from build123d import *

# Parameters (mm, degrees)
F0_W     = 254
F0_H     = 177.8
F1_DEPTH = 1.5875
F2_W     = 1.058418
F2_H     = 63.5
F3_DEPTH = 25.4
F4_R     = 3.96875
F5_DEPTH = 12.7
F6_R     = 3.96875
F7_DEPTH = 12.7


with BuildPart() as f1:
    # F0 (on Top) → F1 (new body)
    with BuildSketch(Plane.XY):
        with Locations((29.202467, -74.189657)):
            Rectangle(F0_W, F0_H)
    extrude(amount=F1_DEPTH)

    # F2 (on face) → F3 (join)
    with BuildSketch(Plane.XY.offset(1.5875)):
        with Locations((118.058609, -74.189657)):
            Rectangle(F2_W, F2_H)
    extrude(amount=F3_DEPTH)

    # F4 (on face) → F5 (join)
    with BuildSketch(Plane.XY.offset(1.5875)):
        with Locations((-34.60809, -83.712486)):
            Circle(F4_R)
        with Locations((-34.8706, -67.839657)):
            Circle(F4_R)
    extrude(amount=F5_DEPTH)

    # F6 (on face) → F7 (join)
    with BuildSketch(Plane.XY.offset(1.5875)):
        with Locations((41.3294, -67.839657)):
            Circle(F6_R)
        with Locations((-34.297533, -151.180522)):
            Circle(F6_R)
    extrude(amount=F7_DEPTH)


solid = f1.part
Geometry: final body of the model. Coordinates: model frame, mm. A direction names the side the tool comes from. Coordinates: 2 decimals unless noted, no trailing zeros. Order: outer loops, then holes, each group sorted by start corner. A loop starts at its lowest first (then second) coordinate and runs counter-clockwise, first axis right, second up.
(1) Section query B-B (y = -55). Return the cut outline in (x, z), plus the area to 3 significant figures.
(2) First-contact query: pin 1 (6.5 mm diameter, centred on x = -35, y = -67, fed in from +Z); pin 2 (7.5 mm diameter, centred on y = -69.5, z = 12, fed in from +X); pin 3 (3 mm diameter, centred on y = -53, z = 21, fed in from -X). Flat tips, straight axial feed; report the tip coordinate or a pass-through.
(3) Material intervals for probe 1 along X at (y, z) = (-84.5, 19.5); probe 2 along Z at (x, y) = (0, -14), sorted ascending.
(4) Section query D-D (z = 18.25). Return the cut outline in (x, y), plus the area to 3 significant figures.
(5) Section query A-A (z = 5.5). Return the cut outline in (x, y), plus the area to 3 significant figures.
(6) Draft query along Y for faces 1 (the face through (40.469, -71.714, 7.849)), 2 (the face through (-37.447, -153.595, 7.849)), 3 (the face through (-34, -151, 14.288)). Return one class per face: pulls with the +Y half, pulls with the -Y half, needs draft (parallel to the pull), parting line crosses it, or undercut.
(7) Access query for faces 4 (the face through (41, -68, 14.288)), 5 (the face through (-35.731, -71.714, 7.849)), 6 (the face through (118.588, -75, 14)), 7 (the face through (117.529, -75, 14)), 8 (the face through (27, -73, 0)). Directions: +Z, -Z, +X, -X, +Y, -Y. A direction counts if a zero-diameter tool reaches every point of the face in a straight line with its end or side. Return the directions, or none.
(8) Section query C-C (x = -27). Return the cut outline in (y, z).
Solution:
1. outline: (-97.8, 0) - (156.2, 0) - (156.2, 1.59) - (118.59, 1.59) - (118.59, 26.99) - (117.53, 26.99) - (117.53, 1.59) - (-97.8, 1.59) - close
1. area: 430 mm2
2. pin 1: stops at z = 14.29
2. pin 2: stops at x = 118.59
2. pin 3: stops at x = 117.53
3. probe 1: x = 117.53 to 118.59
3. probe 2: z = 0 to 1.59
4. outline: (117.53, -105.94) - (118.59, -105.94) - (118.59, -42.44) - (117.53, -42.44) - close
4. area: 67.2 mm2
5. outline: circle Ø7.94 at (-34.87, -67.84); circle Ø7.94 at (-34.61, -83.71); circle Ø7.94 at (-34.3, -151.18); circle Ø7.94 at (41.33, -67.84); (117.53, -105.94) - (118.59, -105.94) - (118.59, -42.44) - (117.53, -42.44) - close
5. area: 265 mm2
6. face 1: parting line crosses it
6. face 2: undercut
6. face 3: needs draft
7. face 4: +Z, -X, +Y, -Y
7. face 5: +Z
7. face 6: +Z, +X, +Y, -Y
7. face 7: +Z, +Y, -Y
7. face 8: -Z, +X, -X, +Y, -Y
8. outline: (-163.09, 0) - (14.71, 0) - (14.71, 1.59) - (-163.09, 1.59) - close
